Study the drawing (mm; zero at the part's minimum x, y, z) and answer. Coordinates: 2 decimals unless noted, no trailing zeros. Loops run counter-clockwise (first coordinate to the right, second up) from the corner with the lowest first, then second, coordinate; pieces in that order, holes last. Notation, with made-up numbers: (82.25, 23.5) - (90.25, 23.5) arc R18 ccw to (90.25, 49.5) - close; hole circle Ø7 at (88, -2.75). An arc over 180 degrees is marked (long way). Use one line per item in the form item = value.
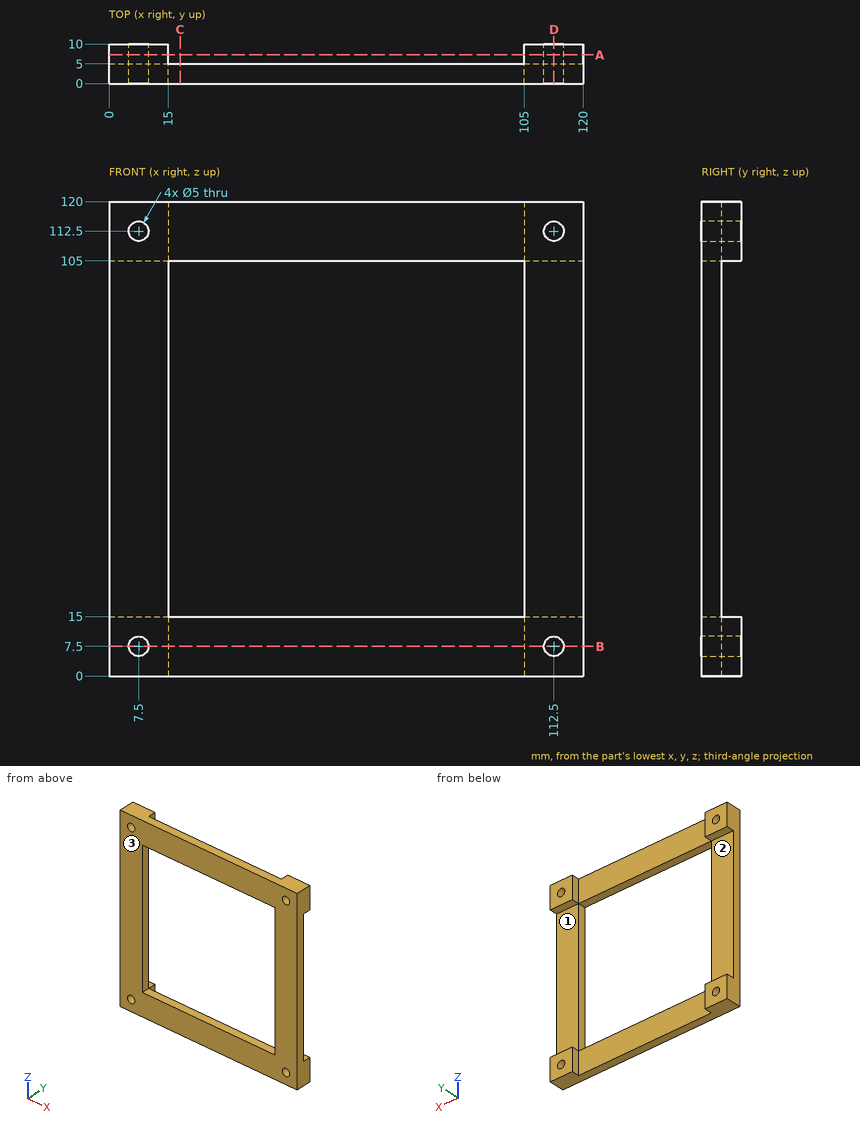
Item 1: The part is cut by section C-C on x = 18. Give the vertices of the cut face in (y, z).
Results below:
outline = (0, 0) - (5, 0) - (5, 15) - (0, 15) - close; (0, 105) - (5, 105) - (5, 120) - (0, 120) - close
Item 2: The part is cut by section A-A on y = 7.25. Give the vertices of the cut face in (x, z).
Results below:
outline = (0, 0) - (15, 0) - (15, 15) - (0, 15) - close; (0, 105) - (15, 105) - (15, 120) - (0, 120) - close; (105, 0) - (120, 0) - (120, 15) - (105, 15) - close; (105, 105) - (120, 105) - (120, 120) - (105, 120) - close; hole circle Ø5 at (7.5, 7.5); hole circle Ø5 at (7.5, 112.5); hole circle Ø5 at (112.5, 7.5); hole circle Ø5 at (112.5, 112.5)
Item 3: This flat-tipped pin is pushed along its axis until it touches: P1, Ø4.5, axis at x = 116, z = 49, coming from the +Y side. Where does it stop, or does it pass through?
Results below:
P1 = 5
Item 4: Find the intervals of material crossed by L1, parallel to Z at x = 112.5, y = 3.5; L2, parallel to X at y = 7, z = 7.5, in increasing order.
Results below:
L1 = 0 to 5, 10 to 110, 115 to 120
L2 = 0 to 5, 10 to 15, 105 to 110, 115 to 120
Item 5: The part is cut by section B-B on z = 7.5. Give the vertices of the cut face in (x, y), plus the area to 3 significant figures.
Results below:
outline = (0, 0) - (5, 0) - (5, 10) - (0, 10) - close; (10, 0) - (110, 0) - (110, 10) - (105, 10) - (105, 5) - (15, 5) - (15, 10) - (10, 10) - close; (115, 0) - (120, 0) - (120, 10) - (115, 10) - close
area = 650 mm²
Item 6: The part is cut by section D-D on x = 112.5. Give the vertices of the cut face in (y, z).
Results below:
outline = (0, 0) - (10, 0) - (10, 5) - (0, 5) - close; (0, 10) - (10, 10) - (10, 15) - (5, 15) - (5, 105) - (10, 105) - (10, 110) - (0, 110) - close; (0, 115) - (10, 115) - (10, 120) - (0, 120) - close
Item 7: For a pull along Z with two mould halves and no side action, classify the marked faces 1, 2 and 3 as +Z half, -Z half, draft (parallel to the pull), parting line (faces both ways), or undercut.
Results below:
face_1 = undercut
face_2 = undercut
face_3 = draft
